Design review of the part built by this model. Coordinates are the model's own, in mm. Coordinates: 2 decimals unless noted, no trailing zeros. Loops run counter-clockwise (first coordinate to the right, second up) from the corner with the lowest first, then second, coordinate; pieces in that order, holes last. Notation, with made-up numbers: (41.25, 72) -> (86.25, 72) arc R24 cw to (86.25, 109) -> close; hole circle Ø10 at (46, 41). An arc over 180 degrees is marked (long way). Answer as a JSON object with one key per item and string values.
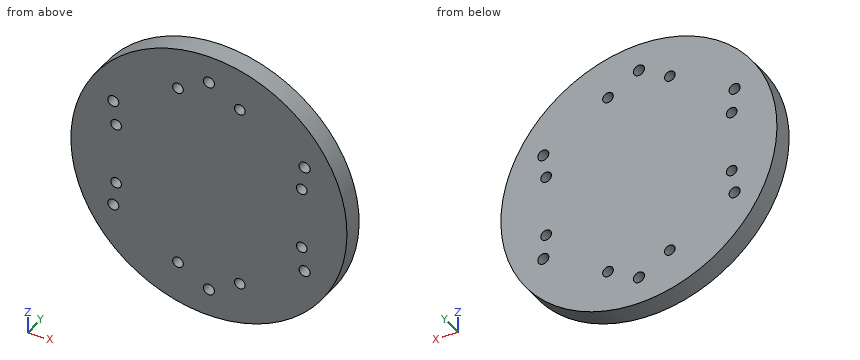
```python
from build123d import *

# Parameters (mm, degrees)
SKETCH1_R                = 85
BOSS_EXTRUDE1_DEPTH      = 12.7
M8X1_25_TAPPED_HOLE1_D   = 6.8
CIRPATTERN3_COUNT        = 6
F_5_16_18_TAPPED_HOLE1_D = 6.5278
CIRPATTERN2_COUNT        = 4


with BuildPart() as part:
    # Sketch1 → Boss-Extrude1 (new body)
    with BuildSketch(Plane(origin=(0, 0, 0), x_dir=(1, 0, 0), z_dir=(0, 1, 0))):
        with Locations(Location((0, 0, 0), (0, 0, 270))):
            Circle(SKETCH1_R)
    extrude(amount=BOSS_EXTRUDE1_DEPTH)

    # M8x1.25 Tapped Hole1 (through all)
    with Locations(Plane(origin=(0, 12.7, 0), x_dir=(1, 0, 0), z_dir=(0, 1, 0))):
        with Locations((0, 68)):
            m8x1_25_tapped_hole1 = Hole(M8X1_25_TAPPED_HOLE1_D / 2)

    # CirPattern3: M8x1.25 Tapped Hole1 ×6 about axis
    cirpattern3_axis = Axis((0, 0, 0), (0, 1, 0))
    for i in range(1, CIRPATTERN3_COUNT):
        add(m8x1_25_tapped_hole1.rotate(cirpattern3_axis, i * 360 / CIRPATTERN3_COUNT), mode=Mode.SUBTRACT)

    # 5/16-18 Tapped Hole1 (through all)
    with Locations(Plane(origin=(0, 0, 0), x_dir=(-1, 0, 0), z_dir=(0, -1, 0))):
        with Locations((-19.049999999, 57.15), (19.049999999, 57.15)):
            f_5_16_18_tapped_hole1 = Hole(F_5_16_18_TAPPED_HOLE1_D / 2)

    # CirPattern2: 5/16-18 Tapped Hole1 ×4 about axis
    cirpattern2_axis = Axis((0, 0, 0), (0, 1, 0))
    for i in range(1, CIRPATTERN2_COUNT):
        add(f_5_16_18_tapped_hole1.rotate(cirpattern2_axis, i * 360 / CIRPATTERN2_COUNT), mode=Mode.SUBTRACT)


solid = part.part
```
1) Add section C-C, the plane y = 2.5. Count the separate pieces of the cut face and the enclosed holes in it, and give its area (3 significant figures).
Completed:
{"separate pieces": "1", "enclosed holes": "14", "area": "22,200 mm²"}
2) Clearance check with flat-ended pins moving along their axes: pin 1 Ø5 at (x, y) = (-14, 2) entering from +Z; pin 2 Ø4 at (x, z) = (58.89, 34) entering from +Y; pin 3 Ø1 at (y, z) = (11, 32) entering from +X; pin 4 Ø5 at (y, z) = (6, -45) entering from +X. State where each tip first meets the part, or that it passes through.
Completed:
{"pin 1": "z = 84.22", "pin 2": "through", "pin 3": "x = 78.95", "pin 4": "x = 73.61"}
3) Add section A-A, the plane z = 68. Give the boundary of the cut face in (x, y).
Completed:
{"outline": "(-51, 0) -> (-3.4, 0) -> (-3.4, 12.7) -> (-51, 12.7) -> close; (3.4, 0) -> (51, 0) -> (51, 12.7) -> (3.4, 12.7) -> close"}
4) Add section B-B, the plane z = -19.05. Give the boundary of the cut face in (x, y), and give its area (3 significant figures).
Completed:
{"outline": "(-82.84, 0) -> (-60.41, 0) -> (-60.41, 12.7) -> (-82.84, 12.7) -> close; (-53.89, 0) -> (53.89, 0) -> (53.89, 12.7) -> (-53.89, 12.7) -> close; (60.41, 0) -> (82.84, 0) -> (82.84, 12.7) -> (60.41, 12.7) -> close", "area": "1,940 mm²"}
5) Add section D-D, the plane x = -36.5. Give the boundary of the cut face in (y, z), and give its area (3 significant figures).
Completed:
{"outline": "(0, -76.76) -> (12.7, -76.76) -> (12.7, 76.76) -> (0, 76.76) -> close", "area": "1,950 mm²"}
6) Wall thickness on probe 1 along X at (y, z) = (7.75, -34); probe 2 along X at (y, z) = (4.5, -19); probe 3 along Z at (x, y) = (-19.5, 6.5): over which ranges is each line inside the solid? List them lowest first.
Completed:
{"probe 1": "-77.9 to -62.29, -55.49 to 55.49, 62.29 to 77.9", "probe 2": "-82.85 to -60.41, -53.89 to 53.89, 60.41 to 82.85", "probe 3": "-82.73 to -60.38, -53.92 to 53.92, 60.38 to 82.73"}
